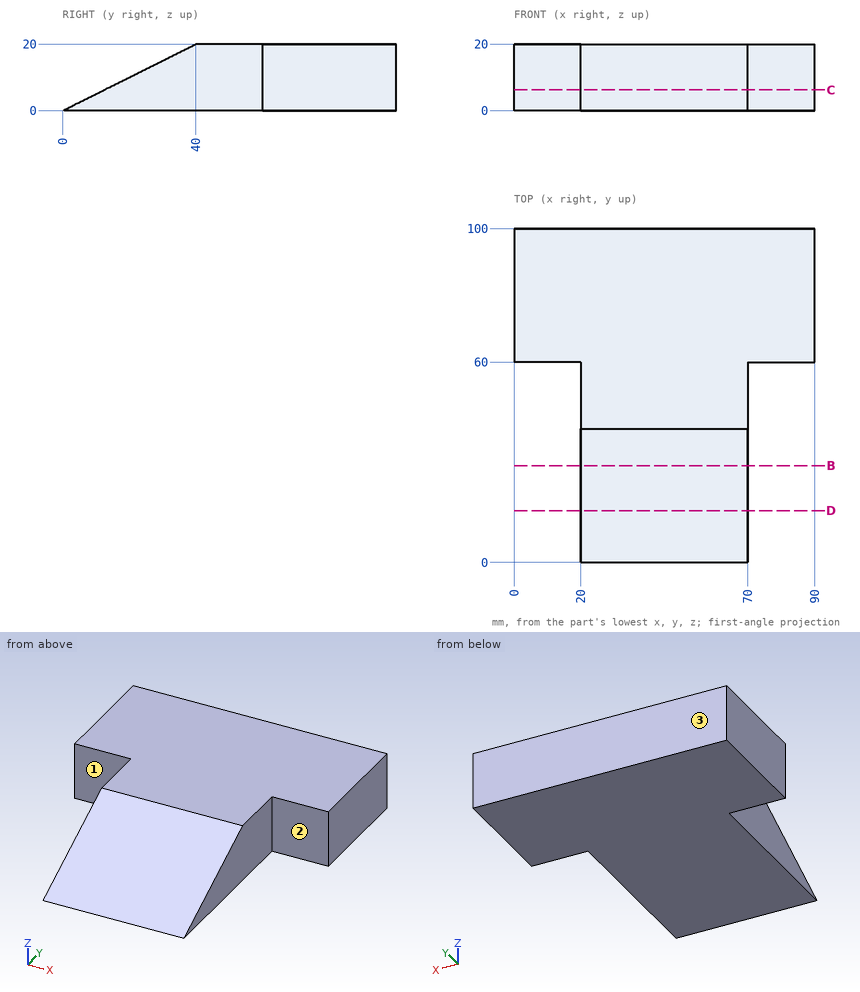
Design review of the part shown in the three views and the two pictorial views. Dimensions are in mm from the part's minimum x, y and z. A direction names the side the tool comes from. Coordinates: 2 decimals unless noted, no trailing zeros. Order: outer loops, then holes, each group sorted by start corner. A loop starts at its lowest first (then second) coordinate and runs counter-clockwise, first axis right, second up. Notation, with made-up numbers: (17, 80.25) - (58, 80.25) arc R16 cw to (58, 87.25) - close; hole circle Ø9 at (-21.5, 74.25). An arc over 180 degrees is marked (long way). Answer as CSV lines item,"result". Start each with the question number.
1) To check wall thickness, follow line 1 along Y through (x, z) = (81, 18.5); line 2 along X through (y, z) = (53.5, 4.5); line 3 along Y through (x, z) = (44, 17.25). State the ranges of each line that lie inside material, in increasing order. Write a range as [from, to].
2) Insertion check: P1, Ø6, axis at x = 23.5, z = 3.5, coming from the -Y side; P2, Ø1, axis at x = 50, z = 12, coming from the -Y side; P3, Ø6, axis at y = 32.5, z = 13, coming from the +X side. Each pin has a flat end and moves straight along its axis. Give the tip position at first contact, or say it passes through.
3) Add section C-C (z = 6.25). State the section outline as (x, y) points.
4) Add section B-B (y = 29). State the section outline as (x, z) points.
5) Add section D-D (y = 15.5). State the section outline as (x, z) points.
6) Machinability: for the marked faces 1, 2 and 3, which of the approach directions +Z, -Z, +X, -X, +Y, -Y give a long, thin tool a straight path to every point of the face, cutting with its end or side? Answer none if there is none.
Result:
1,line 1,"[60, 100]"
1,line 2,"[20, 70]"
1,line 3,"[34.5, 100]"
2,P1,"y = 1"
2,P2,"y = 23"
2,P3,"x = 70"
3,outline,"(0, 60) - (20, 60) - (20, 12.5) - (70, 12.5) - (70, 60) - (90, 60) - (90, 100) - (0, 100) - close"
4,outline,"(20, 0) - (70, 0) - (70, 14.5) - (20, 14.5) - close"
5,outline,"(20, 0) - (70, 0) - (70, 7.75) - (20, 7.75) - close"
6,face 1,"+Z, -Z, -X, -Y"
6,face 2,"+Z, -Z, +X, -Y"
6,face 3,"+Z, -Z, +X, -X, +Y"
